Input: part model. Units: mm. Frame: model coordinates. A direction names the side the tool comes from. Round coordinates to 2 decimals unless told otherwise and drop trailing zeros. Order: outer loops, then holes, each group sorted by start corner. A loop starts at its lowest first (then second) coordinate and runs counter-clockwise, first axis right, second up.
Item 1: Cut plane D-D on y = -16. Output: boundary loops of the cut face in (x, z), then the cut area to 3 significant figures.
Item 2: Reachability of faces 4 (the flat face through (-61, -4.311, 3)), 5 (the cylindrical face through (-33.155, 0.072, 2.958)) from +Z, -Z, +X, -X, +Y, -Y: full face, straight path, thin tool, end or side. Return the list, or none.
Item 3: Mould query, pull axis Y, two halves, no side actions, for faces 1 (the cylindrical face through (-49.207, -0.454, 2.958)), 2 (the flat face through (-180, 19.632, 3)), 3 (the flat face through (-176, -20.368, 3)). Classes: released by +Y, released by -Y, zero draft, split by the parting line, or undercut.
Item 4: First-contact query: pin 1 (1 mm diameter, centred on y = 4.5, z = 2, fed in from +X); pin 2 (2 mm diameter, centred on y = 0.5, z = 5.5, fed in from +X). Flat tips, straight axial feed; report the tip coordinate or a pass-through.
Item 5: Cut plane A-A on x = -59.5. Output: boundary loops of the cut face in (y, z), then the cut area to 3 significant figures.
Item 6: Cut plane C-C on y = -1. Output: boundary loops of the cut face in (x, z).
Item 7: Line query: L1, parallel to X at y = -0.5, z = 1.5; L2, parallel to Y at x = -53, z = 4.4; L3, parallel to X at y = -2, z = 0.6. Output: solid intervals per line, ascending.
Item 8: Cut plane B-B on z = 4.1. Output: boundary loops of the cut face in (x, y).
```python
from build123d import *

# Parameters (mm, degrees)
BOSS_EXTRUDE1_DEPTH = 6
CUT_EXTRUDE1_REACH  = 8


with BuildPart() as part:
    # Sketch1 → Boss-Extrude1 (new body)
    with BuildSketch(Plane.XY):
        with BuildLine():
            Line((-53.14999664, -20.367507575), (-303.15, -20.367507575))
            ThreePointArc((-303.15, -20.367507575), (-323.15, -0.367507575), (-303.15, 19.632492425))
            Line((-303.15, 19.632492425), (-53.14999664, 19.632492425))
            ThreePointArc((-53.14999664, 19.632492425), (-33.15, -0.367507575), (-53.14999664, -20.367507575))
        make_face()
    extrude(amount=BOSS_EXTRUDE1_DEPTH)

    # Sketch2 → Cut-Extrude1 (cut, up to next)
    with BuildSketch(Plane(origin=(0, 0, 0), x_dir=(-1, 0, 0), z_dir=(0, 0, -1)), mode=Mode.PRIVATE) as cut_extrude1_sk1:
        with BuildLine():
            Line((53.15, 3.576263022), (68.15, 3.576263022))
            ThreePointArc((68.15, 3.576263022), (72.093770597, -0.367507575), (68.15, -4.311278172))
            Line((68.15, -4.311278172), (53.15, -4.311278172))
            ThreePointArc((53.15, -4.311278172), (49.206229403, -0.367507575), (53.15, 3.576263022))
        make_face()
    cut_extrude1_tool1 = extrude(cut_extrude1_sk1.sketch, amount=-CUT_EXTRUDE1_REACH, mode=Mode.PRIVATE) & part.part
    add(cut_extrude1_tool1.solids().sort_by_distance((-60.65, -0.367508, 0))[0], mode=Mode.SUBTRACT)


solid = part.part
```
From the geometry:
1. outline: (-315.62, 0) - (-40.68, 0) - (-40.68, 6) - (-315.62, 6) - close
1. area: 1,650 mm2
2. face 4: +Z, -Z
2. face 5: +Z, -Z, +X
3. face 1: undercut
3. face 2: released by +Y
3. face 3: released by -Y
4. pin 1: stops at x = -33.63
4. pin 2: stops at x = -33.15
5. outline: (-20.37, 0) - (-4.31, 0) - (-4.31, 6) - (-20.37, 6) - close; (3.58, 0) - (19.63, 0) - (19.63, 6) - (3.58, 6) - close
5. area: 193 mm2
6. outline: (-323.14, 0) - (-72.04, 0) - (-72.04, 6) - (-323.14, 6) - close; (-49.26, 0) - (-33.16, 0) - (-33.16, 6) - (-49.26, 6) - close
7. L1: x = -323.15 to -72.09, -49.21 to -33.15
7. L2: y = -20.37 to -4.31, 3.57 to 19.63
7. L3: x = -323.08 to -71.74, -49.56 to -33.22
8. outline: (-303.15, -20.37) - (-53.15, -20.37) arc R20 ccw to (-53.15, 19.63) - (-303.15, 19.63) arc R20 ccw to start; hole (-68.15, -4.31) - (-53.15, -4.31) arc R3.94 ccw to (-53.15, 3.58) - (-68.15, 3.58) arc R3.94 ccw to start
